Part model, mm, in its own coordinate system. Give positions to 0.01 mm unless a question says otherwise; leave off trailing zeros. Write each loop counter-clockwise with the first axis right and the second up, starting at its lowest first coordinate (ties: lowest second). Pieces come first, ordered by that corner, then holes. Notation, with made-up numbers: M -21,83.5 L 38,83.5 A31 ccw 38,107.5 Z; hole C -4.5,-29 d2. An arc over 180 degrees is marked long. Use a Markdown table: item, result.
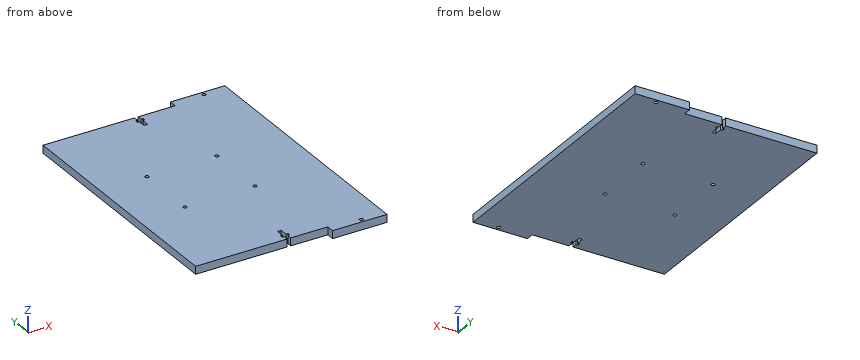
```python
from build123d import *

# Parameters (mm, degrees)
BOSS_EXTRUDE1_DEPTH = 6.35
SKETCH2_R           = 1.4732
CUT_EXTRUDE1_DEPTH  = 265.346160366
SKETCH4_R           = 1.524
CUT_EXTRUDE2_DEPTH  = 265.346160366
SKETCH5_R           = 1.524
CUT_EXTRUDE3_DEPTH  = 265.346160366
CUT_EXTRUDE10_DEPTH = 265.346160366


with BuildPart() as part:
    # Sketch1 → Boss-Extrude1 (new body)
    with BuildSketch(Plane.XY):
        Polygon((107.95, 215.9), (107.95, 209.55), (0, 209.55), (0, 6.35), (107.95, 6.35), (107.95, 0), (152.4, 0), (152.4, 215.9), align=None)
    extrude(amount=BOSS_EXTRUDE1_DEPTH)

    # Sketch2 → Cut-Extrude1 (cut, through all)
    with BuildSketch(Plane.XY.offset(6.35)):
        with Locations(Location((133.35, 212.725, 0), (0, 0, 180))):
            Circle(SKETCH2_R)
        with Locations((133.35, 3.175)):
            Circle(SKETCH2_R)
    extrude(amount=-CUT_EXTRUDE1_DEPTH, mode=Mode.SUBTRACT)

    # Sketch4 → Cut-Extrude2 (cut, through all)
    with BuildSketch(Plane.XY.offset(6.35)):
        with Locations(Location((95.25, 133.35, 0), (0, 0, 180))):
            Circle(SKETCH4_R)
        with Locations((95.25, 82.55)):
            Circle(SKETCH4_R)
    extrude(amount=-CUT_EXTRUDE2_DEPTH, mode=Mode.SUBTRACT)

    # Sketch5 → Cut-Extrude3 (cut, through all)
    with BuildSketch(Plane.XY.offset(6.35)):
        with Locations((38.1, 133.35)):
            Circle(SKETCH5_R)
        with Locations(Location((38.1, 82.55, 0), (0, 0, 180))):
            Circle(SKETCH5_R)
    extrude(amount=-CUT_EXTRUDE3_DEPTH, mode=Mode.SUBTRACT)

    # Sketch10 → Cut-Extrude10 (cut, through all)
    with BuildSketch(Plane(origin=(0, 0, 0), x_dir=(-1, 0, 0), z_dir=(0, 0, -1))):
        Polygon((-77.6732, 6.35), (-74.7268, 6.35), (-74.7268, 10.31875), (-73.025, 10.31875), (-73.025, 12.7), (-74.7268, 12.7), (-74.7268, 19.05), (-77.6732, 19.05), (-77.6732, 12.7), (-79.375, 12.7), (-79.375, 10.31875), (-77.6732, 10.31875), align=None)
        Polygon((-73.025, 205.58125), (-73.025, 203.2), (-74.7268, 203.2), (-74.7268, 196.85), (-77.6732, 196.85), (-77.6732, 203.2), (-79.375, 203.2), (-79.375, 205.58125), (-77.6732, 205.58125), (-77.6732, 209.55), (-74.7268, 209.55), (-74.7268, 205.58125), align=None)
    extrude(amount=-CUT_EXTRUDE10_DEPTH, mode=Mode.SUBTRACT)


solid = part.part
```
1. Cut at B-B, the plane z = 4.75. State how many separate pieces and enclosed holes the cut face has, then the cut area to 3 significant figures.
Findings below:
| item | result |
|---|---|
| separate pieces | 1 |
| enclosed holes | 6 |
| area | 31,400 mm2 |
2. Drop flat-ended pins along their axis: P1, Ø1.9, axis at x = 78.5, z = 3, coming from the -Y side; P2, Ø2.5, axis at x = 133.35, y = 3.175, coming from the +Z side; P3, Ø3, axis at y = 213.5, z = 3, coming from the -X side; P4, Ø2.5, axis at x = 76.5, z = 2, coming from the +Y side. Give the stop position or say it passes through.
Findings below:
| item | result |
|---|---|
| P1 | y = 6.35 |
| P2 | through |
| P3 | x = 107.95 |
| P4 | y = 209.55 |
3. Cut at A-A, the plane x = 57. Give the cut face in (y, z).
Findings below:
| item | result |
|---|---|
| outline | M 6.35,0 L 209.55,0 L 209.55,6.35 L 6.35,6.35 Z |
4. Drill centre lines: L1, parallel to Y at x = 133, z = 3.25; L2, parallel to X at y = 133.35, z = 4; L3, parallel to Y at x = 38.1, z = 2. Where is each one in solid material? Low to high.
Findings below:
| item | result |
|---|---|
| L1 | 0 to 1.74, 4.61 to 211.29, 214.16 to 215.9 |
| L2 | 0 to 36.58, 39.62 to 93.73, 96.77 to 152.4 |
| L3 | 6.35 to 81.03, 84.07 to 131.83, 134.87 to 209.55 |
